Geometry: final body of the model. Coordinates: model frame, mm. A direction names the side the tool comes from. Coordinates: 2 decimals unless noted, no trailing zeros. Write each loop counter-clockwise with the first axis right and the second up, starting at its lowest first coordinate (ties: lowest second). Pieces come first, ordered by that corner, then holes. Notation, with made-up numbers: (58, 54) - (103, 54) arc R18 cw to (103, 82) - close; hole circle Ø10 at (9, 68). An arc over 180 degrees is marked (long way). Answer as a JSON object with one key per item and string values. Group by question number.
Item 1: Section B-B on x = -47.5. Return loops of the section in (y, z).
Item 2: Section A-A on z = -66.25. Return loops of the section in (x, y).
Item 3: Line query: line 1 along Z through (x, y) = (-47.5, 1.25); line 2 along X through (y, z) = (1.05, 66.25); line 3 along Y through (x, z) = (-34, 0.5). Output: solid intervals per line, ascending. Write a range as from..to.
Item 4: Set-up query: faces 1 (the flat face through (1, 1.75, 66)), 2 (the flat face through (-10.97, -3, -65)), 3 (the flat face through (1, 1.75, -66)), 4 (the flat face through (9.03, -3, -65)). Return all of +Z, -Z, +X, -X, +Y, -Y with unobstructed straight access to the full face (end or side cutting, diameter ignored); none if empty.
Item 5: Mould query, pull axis Z, two halves, no side actions, for faces 5 (the flat face through (-1, -6, -65)), 6 (the cylindrical face through (-49, 0.9, 66.2)), 7 (the flat face through (-1, -3, -61.4)), 8 (the cylindrical face through (-49, 0.9, -66.3)). Classes: pulls with the +Z half, pulls with the -Z half, needs draft (parallel to the pull), parting line crosses it, or undercut.
Item 6: First-contact query: pin 1 Ø5.5 at (x, z) = (21.5, 67.5) entering from +Y; pin 2 Ø8 at (x, z) = (-4, -44.5) entering from -Y; pin 3 Ø5 at (x, y) = (-0.5, -4) entering from +Z. Flat tips, straight axial feed; report the tip coordinate or a pass-through.
Autodesk Inventor part; units mm, degrees
ref_plane "YZ Plane" through (0, 0, 0) normal (1, 0, 0) x (0, 1, 0)
ref_plane "XZ Plane" through (0, 0, 0) normal (0, 1, 0) x (-1, 0, 0)
ref_plane "XY Plane" through (0, 0, 0) normal (0, 0, 1) x (1, 0, 0)
sketch "Sketch1" plane through (0, 0, 0) normal (0, 1, 0) x (-1, 0, 0)
  line L0 (-50.22, 69.4) -> (50.22, 69.4)
  line L1 (50.22, 69.4) -> (50.22, -69.4)
  line L2 (50.22, -69.4) -> (-50.22, -69.4)
  line L3 (-50.22, -69.4) -> (-50.22, 69.4)
  line L4 (-50.22, 69.4) -> (50.22, -69.4) construction
  line L5 (50.22, 69.4) -> (-50.22, -69.4) construction
  point P0 (0, 0)
  dimension "d0" = 100.44
  dimension "d1" = 138.8
extrude "Extrusion1" add sketch "Sketch1" along normal blind 1.75
sketch "Sketch2" plane through (0, 1.75, 0) normal (0, 1, 0) x (1, 0, 0)
  line L0 (-50.22, 69.4) -> (-50.22, -69.4) construction
  line L1 (50.22, -69.4) -> (50.22, 69.4) construction
  line L2 (50.22, -62.5) -> (-50.22, -62.5)
  line L3 (-50.22, -62.5) -> (-50.22, 62.5)
  line L4 (-50.22, 62.5) -> (50.22, 62.5)
  line L5 (50.22, 62.5) -> (50.22, -62.5)
  line L6 (50.22, -62.5) -> (-50.22, 62.5) construction
  line L7 (-50.22, -62.5) -> (50.22, 62.5) construction
  point P0 (0, 0)
  dimension "d4" = 125
extrude "Extrusion2" add sketch "Sketch2" along normal blind 1.75
sketch "Sketch3" plane through (0, 1.75, 0) normal (0, 1, 0) x (1, 0, 0)
  line L0 (50.22, -62.5) -> (-50.22, -62.5) construction
  line L1 (-50.22, -62.5) -> (-50.22, -69.4) construction
  line L2 (-50.22, -69.4) -> (50.22, -69.4) construction
  line L3 (50.22, -69.4) -> (50.22, -62.5) construction
  line L4 (-50.22, 62.5) -> (50.22, 62.5) construction
  line L5 (50.22, 62.5) -> (50.22, 69.4) construction
  line L6 (50.22, 69.4) -> (-50.22, 69.4) construction
  line L7 (-50.22, 69.4) -> (-50.22, 62.5) construction
  line L8 (-50.22, -69.4) -> (50.22, -69.4) construction
  line L9 (0, -69.4) -> (0, 69.4) construction
  line L10 (50.22, 69.4) -> (-50.22, 69.4) construction
  line L11 (0, -66.25) -> (-47.5, -66.25) construction
  line L12 (0, -66.25) -> (47.5, -66.25) construction
  line L13 (-50.22, -62.5) -> (50.22, -62.5) construction
  line L14 (0, -66.25) -> (47.5, -66.25) construction
  circle A0 centre (-47.5, -66.25) radius 1.5
  circle A1 centre (47.5, -66.25) radius 1.5
  line L15 (-50.22, 69.4) -> (-50.22, -69.4)
  line L16 (-50.22, 0) -> (50.22, 0) construction
  line L17 (50.22, -62.5) -> (50.22, 62.5)
  circle A2 centre (-47.5, 66.25) radius 1.5
  circle A3 centre (47.5, 66.25) radius 1.5
  line L18 (50.22, -62.5) -> (-50.22, -62.5)
  line L19 (-50.22, -62.5) -> (-50.22, -69.4)
  line L20 (-50.22, -69.4) -> (50.22, -69.4)
  line L21 (50.22, -69.4) -> (50.22, -62.5)
  line L22 (-50.22, 62.5) -> (50.22, 62.5)
  line L23 (50.22, 69.4) -> (-50.22, 69.4)
  line L24 (50.22, 62.5) -> (50.22, 69.4)
  line L25 (-50.22, 69.4) -> (-50.22, 62.5)
  point P0 (0, 0)
  point P1 (-51, 62.5)
  dimension "d7" = 47.5
  dimension "d8" = 47.5
  dimension "d9" = 0
  dimension "d10" = 3
  dimension "d11" = 3
extrude "Extrusion3" cut sketch "Sketch3" against normal through all contours A0 | A1 | A2 | A3
sketch "Sketch4" plane through (0, 0, 0) normal (0, -1, 0) x (1, 0, 0)
  circle A0 centre (47.5, -66.25) radius 1.5 construction
  circle A1 centre (-47.5, -66.25) radius 1.5 construction
  circle A2 centre (47.5, 66.25) radius 1.5 construction
  circle A3 centre (-47.5, 66.25) radius 1.5 construction
  line L0 (-50.22, 69.4) -> (50.22, 69.4) construction
  line L1 (-50.22, -69.4) -> (-50.22, 69.4) construction
  line L2 (50.22, -69.4) -> (-50.22, -69.4) construction
  line L3 (50.22, 69.4) -> (50.22, -69.4) construction
  circle A4 centre (-47.5, -66.25) radius 1.5 construction
  line L4 (50.22, -69.4) -> (8.97, -69.4) construction
  line L5 (50.22, -69.4) -> (-50.22, -69.4) construction
  line L6 (-50.22, -69.4) -> (-10.97, -69.4) construction
  line L7 (-10.97, -69.4) -> (-10.97, -61.4)
  line L8 (-10.97, -61.4) -> (9.03, -61.4)
  line L9 (9.03, -61.4) -> (9.03, -69.4)
  line L10 (9.03, -69.4) -> (-10.97, -69.4)
  point P0 (0, 0)
  dimension "d21" = 41.25
  dimension "d22" = 39.25
  dimension "d23" = 8
  dimension "d24" = 20
extrude "Extrusion4" add sketch "Sketch4" along normal blind 6
sketch "Sketch5" plane through (0, 3.5, 0) normal (0, 1, 0) x (1, 0, 0)
  line L0 (50.22, 62.5) -> (-50.22, 62.5) construction
  line L1 (-50.22, 62.5) -> (-50.22, -62.5) construction
  line L2 (-50.22, -62.5) -> (50.22, -62.5) construction
  line L3 (50.22, -62.5) -> (50.22, 62.5) construction
  line L4 (-50.22, 62.5) -> (-50.22, -62.5) construction
  line L5 (-50.22, 62.5) -> (-50.22, 55.388) construction
  line L6 (-50.22, 55.388) -> (-43.108, 55.388) construction
  line L7 (50.22, 62.5) -> (50.22, 55.388) construction
  line L8 (50.22, -62.5) -> (50.22, 62.5) construction
  line L9 (50.22, 55.388) -> (41.33, 55.388) construction
  line L10 (-50.22, -62.5) -> (50.22, -62.5) construction
  line L11 (50.22, -62.5) -> (50.22, -55.388) construction
  line L12 (50.22, -55.388) -> (41.33, -55.388) construction
  line L13 (-50.22, -62.5) -> (-50.22, -69.4) construction
  line L14 (-50.22, -62.5) -> (-50.22, -55.388) construction
  line L15 (-50.22, -55.388) -> (-43.108, -55.388) construction
  line L16 (-43.108, 55.388) -> (45.775, 55.388)
  line L17 (45.775, 55.388) -> (45.775, -55.388)
  line L18 (45.775, -55.388) -> (-43.108, -55.388)
  line L19 (-43.108, -55.388) -> (-43.108, 55.388)
  point P0 (0, 0)
  dimension "d25" = 7.112
  dimension "d26" = 7.112
  dimension "d27" = 7.112
  dimension "d28" = 8.89
  dimension "d29" = 7.112
  dimension "d30" = 8.89
  dimension "d31" = 7.112
  dimension "d32" = 7.112
extrude "Extrusion5" add sketch "Sketch5" along normal blind 0.001
equation "\"d26\" = d25"
equation "\"d27\" = d25"
equation "\"d29\" = d25"
equation "\"d30\" = d28"
equation "\"d31\" = d25"
equation "\"d32\" = d25"
properties part number "E-Paper Display"
Checks:
{
 "1": {"outline": "(0, -69.4) - (1.75, -69.4) - (1.75, -67.75) - (0, -67.75) - close; (0, -64.75) - (1.75, -64.75) - (1.75, -62.5) - (3.5, -62.5) - (3.5, 62.5) - (1.75, 62.5) - (1.75, 64.75) - (0, 64.75) - close; (0, 67.75) - (1.75, 67.75) - (1.75, 69.4) - (0, 69.4) - close"},
 "2": {"outline": "(-50.22, 0) - (-49, 0) - (-49, 1.75) - (-50.22, 1.75) - close; (-46, 0) - (-10.97, 0) - (-10.97, -6) - (9.03, -6) - (9.03, 0) - (46, 0) - (46, 1.75) - (-46, 1.75) - close; (49, 0) - (50.22, 0) - (50.22, 1.75) - (49, 1.75) - close"},
 "3": {"line 1": "-69.4..-67.75, -64.75..64.75, 67.75..69.4", "line 2": "-50.22..-49, -46..46, 49..50.22", "line 3": "0..3.5"},
 "4": {"face 1": "+Z, +X, -X, +Y", "face 2": "+Z, -Z, -X, -Y", "face 3": "-Z, +X, -X, +Y", "face 4": "+Z, -Z, +X, -Y"},
 "5": {"face 5": "needs draft", "face 6": "undercut", "face 7": "pulls with the +Z half", "face 8": "undercut"},
 "6": {"pin 1": "y = 1.75", "pin 2": "y = 0", "pin 3": "z = -61.4"}
}
